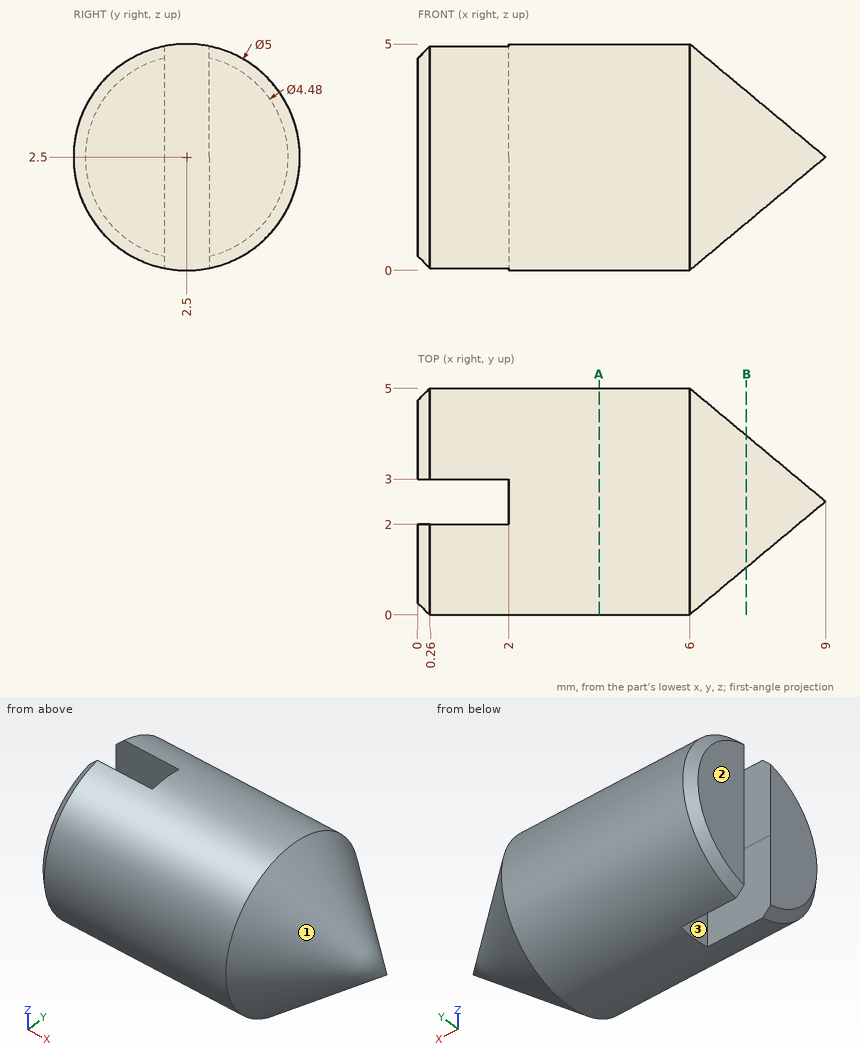
Check sheet for the drawn part. Datum: minimum x, y, z corner. Units: mm. Round coordinates to 2 decimals unless told otherwise and drop trailing zeros. Order: outer loops, then holes, each group sorted by start corner. A loop starts at its lowest first (then second) coordinate and runs counter-clockwise, first axis right, second up. Notation, with made-up numbers: (27, 0) - (35, 0) arc R30 ccw to (35, 39) - close; hole circle Ø11 at (17.5, -34). An arc over 180 degrees is marked (long way). Use a Markdown table: item, result. Add a question column.
(1) Depth check by flat-ended pin: pin 1 (1 mm diameter, centred on y = 3.5, z = 2, fed in from +X); pin 2 (1.6 mm diameter, centred on x = 0.5, z = 1, fed in from -Y); pin 3 (1.6 mm diameter, centred on x = 1.5, z = 1, fed in from +Y). Enter the tip coordinate at first touch or a pass-through.
(2) Sectioned sample at A-A, the plane x = 4. Enter the section's corners in (y, z), and give its area (3 significant figures).
(3) Release check for a two-part mould opening along Y. For the marked faces 1, 2 and 3 record: pulls with the +Y half, pulls with the -Y half, needs draft (parallel to the pull), parting line crosses it, or undercut.
(4) Material ranges on line 1 along Y through (x, z) = (1.25, 1.3); line 2 along Z through (x, y) = (4.75, 0.35); line 3 along X through (y, z) = (1.25, 2.2), recorded low to high. Write a range as [from, to].
(5) Sectioned sample at B-B, the plane x = 7.25. Enter the section's corners in (y, z), and give its area (3 significant figures).
Answers below:
| question | item | result |
|---|---|---|
| 1 | pin 1 | x = 8.26 |
| 1 | pin 2 | y = 0.1 |
| 1 | pin 3 | y = 4.9 |
| 2 | outline | circle Ø5 at (2.5, 2.5) |
| 2 | area | 19.6 mm² |
| 3 | face 1 | parting line crosses it |
| 3 | face 2 | needs draft |
| 3 | face 3 | undercut |
| 4 | line 1 | [0.31, 2], [3, 4.69] |
| 4 | line 2 | [1.22, 3.78] |
| 4 | line 3 | [0, 7.46] |
| 5 | outline | circle Ø2.92 at (2.5, 2.5) |
| 5 | area | 6.68 mm² |
